The model under review builds one solid part; all positions refer to its coordinate system, in mm. A direction names the side the tool comes from. Round coordinates to 2 decimals unless told otherwise and drop trailing zeros. Write each loop counter-clockwise with the first axis right and the second up, starting at its lowest first coordinate (ties: lowest second). Pieces come first, ordered by that corner, then holes. Notation, with made-up numbers: M 3.5,-28.5 L 42.5,-28.5 A31 ccw 42.5,8.5 Z; hole C 4,32 d7. An arc over 180 degrees is marked long. One line per item, written item: value. Start each with the question number.
1) Wall thickness on probe 1 along Y at (x, z) = (13, 0.8); probe 2 along X at (y, z) = (-21.5, 1.15); probe 3 along Y at (x, z) = (-15, 0.25): over which ranges is each line inside the solid? List them lowest first.
2) For P1, Ø0.6, axis at x = -3.5, z = 1, coming from the -Y side; P2, Ø1, axis at x = -3.5, z = 1, coming from the +Y side, all flat-tipped, find the tip position at first contact; note any pin that passes through.
3) Mouldability with a two-part tool opening along X and no side actions: class faces 1 (the face through (3, -2, 0)), 2 (the face through (-16.55, -6.49, 0.99)), 3 (the face through (22.039, -6.507, 0.986)), 4 (the face through (-4.946, 17.079, 1.014)) as +X half, -X half, draft (parallel to the pull), parting line (faces both ways), or undercut.
4) Take a section at A-A, the plane x = -7.5. Write out the cut boundary in (y, z).
5) Take a section at D-D, the plane x = -15. Write out the cut boundary in (y, z).
6) Tool access review of faces 5 (the face through (9, 16.794, 1)), 6 (the face through (-16.246, 4, 1)), 7 (the face through (9, -21.206, 1)): name each direction out of +Z, -Z, +X, -X, +Y, -Y from which nothing blocks a thin tool from reaching the whole face with its end or side.
7) Take a section at C-C, the plane z = 1.05. State how many separate pieces and enclosed holes the cut face has, and give its area (3 significant figures).
8) Take a section at B-B, the plane x = 20.5. Write out the cut boundary in (y, z).
from build123d import *

# Parameters (mm, degrees)
SKETCH_1_R          = 1
EXTRUDE_4_DEPTH     = 2
FILLET_1_R          = 1
EXTRUDE_5_DEPTH     = 2
SKETCH_5_R          = 1
CUT_EXTRUDE_3_DEPTH = 2
SKETCH_6_W          = 8
SKETCH_6_H          = 3
EXTRUDE_6_DEPTH     = 2


with BuildPart() as part:
    # 草圖1 → 填料-伸長4 (new body)
    with BuildSketch(Plane.XY):
        with BuildLine():
            Line((-19.246232324, 5.793640832), (-17.246232324, 5.793640832))
            ThreePointArc((-17.246232324, 5.793640832), (-16.539125543, 5.500747613), (-16.246232324, 4.793640832))
            Line((-16.246232324, 4.793640832), (-16.246232324, 2.793640832))
            ThreePointArc((-16.246232324, 2.793640832), (-16.539125543, 2.086534051), (-17.246232324, 1.793640832))
            Line((-17.246232324, 1.793640832), (-19.246232324, 1.793640832))
            Line((-19.246232324, 1.793640832), (-19.246232324, -6.206359168))
            Line((-19.246232324, -6.206359168), (-17.246232324, -6.206359168))
            ThreePointArc((-17.246232324, -6.206359168), (-16.539125543, -6.499252387), (-16.246232324, -7.206359168))
            Line((-16.246232324, -7.206359168), (-16.246232324, -9.206359168))
            ThreePointArc((-16.246232324, -9.206359168), (-16.539125543, -9.913465949), (-17.246232324, -10.206359168))
            Line((-17.246232324, -10.206359168), (-19.246232324, -10.206359168))
            Line((-19.246232324, -10.206359168), (-19.246232324, -18.206359168))
            Line((-19.246232324, -18.206359168), (24.753767676, -18.206359168))
            Line((24.753767676, -18.206359168), (24.753767676, -10.206359168))
            Line((24.753767676, -10.206359168), (22.753767676, -10.206359168))
            ThreePointArc((22.753767676, -10.206359168), (22.046660894, -9.913465949), (21.753767676, -9.206359168))
            Line((21.753767676, -9.206359168), (21.753767676, -7.206359168))
            ThreePointArc((21.753767676, -7.206359168), (22.046660894, -6.499252387), (22.753767676, -6.206359168))
            Line((22.753767676, -6.206359168), (24.753767676, -6.206359168))
            Line((24.753767676, -6.206359168), (24.753767676, 1.793640832))
            Line((24.753767676, 1.793640832), (22.753767676, 1.793640832))
            ThreePointArc((22.753767676, 1.793640832), (22.046660894, 2.086534051), (21.753767676, 2.793640832))
            Line((21.753767676, 2.793640832), (21.753767676, 4.793640832))
            ThreePointArc((21.753767676, 4.793640832), (22.046660894, 5.500747613), (22.753767676, 5.793640832))
            Line((22.753767676, 5.793640832), (24.753767676, 5.793640832))
            Line((24.753767676, 5.793640832), (24.753767676, 13.793640832))
            Line((24.753767676, 13.793640832), (-19.246232324, 13.793640832))
            Line((-19.246232324, 13.793640832), (-19.246232324, 5.793640832))
        make_face()
        with Locations((-15.246232324, 7.793640832)):
            Circle(SKETCH_1_R, mode=Mode.SUBTRACT)
        with Locations((-15.246232324, -0.206359168)):
            Circle(SKETCH_1_R, mode=Mode.SUBTRACT)
        with Locations((20.753767676, -12.206359168)):
            Circle(SKETCH_1_R, mode=Mode.SUBTRACT)
        with Locations((20.753767676, 7.793640832)):
            Circle(SKETCH_1_R, mode=Mode.SUBTRACT)
        with Locations((-15.246232324, -4.206359168)):
            Circle(SKETCH_1_R, mode=Mode.SUBTRACT)
        with Locations((-15.246232324, -12.206359168)):
            Circle(SKETCH_1_R, mode=Mode.SUBTRACT)
        with Locations((20.753767676, -0.206359168)):
            Circle(SKETCH_1_R, mode=Mode.SUBTRACT)
        with Locations((20.753767676, -4.206359168)):
            Circle(SKETCH_1_R, mode=Mode.SUBTRACT)
    extrude(amount=EXTRUDE_4_DEPTH)

    # 圓角1
    fillet_1_edges = [part.edges().sort_by_distance(p)[0] for p in [
        (-19.246232324, 13.793640832, 1),
        (24.753767676, 13.793640832, 1),
        (24.753767676, -18.206359168, 1),
        (-19.246232324, -18.206359168, 1),
    ]]
    fillet(fillet_1_edges, radius=FILLET_1_R)

    # 草圖4 → 填料-伸長5 (add)
    with BuildSketch(Plane.XY.offset(2)):
        with BuildLine():
            Line((-19.246232324, -21.206359168), (-19.246232324, -17.206359168))
            Line((-19.246232324, -17.206359168), (24.753767676, -17.206359168))
            Line((24.753767676, -17.206359168), (24.753767676, -21.206359168))
            ThreePointArc((24.753767676, -21.206359168), (24.460874457, -21.913465949), (23.753767676, -22.206359168))
            Line((23.753767676, -22.206359168), (-18.246232324, -22.206359168))
            ThreePointArc((-18.246232324, -22.206359168), (-18.953339106, -21.913465949), (-19.246232324, -21.206359168))
        make_face()
        with BuildLine():
            Line((-19.246232324, 12.793640832), (24.753767676, 12.793640832))
            Line((24.753767676, 12.793640832), (24.753767676, 16.793640832))
            ThreePointArc((24.753767676, 16.793640832), (24.460874457, 17.500747613), (23.753767676, 17.793640832))
            Line((23.753767676, 17.793640832), (-18.246232324, 17.793640832))
            ThreePointArc((-18.246232324, 17.793640832), (-18.953339106, 17.500747613), (-19.246232324, 16.793640832))
            Line((-19.246232324, 16.793640832), (-19.246232324, 12.793640832))
        make_face()
    extrude(amount=-EXTRUDE_5_DEPTH)

    # 草圖5 → 除料-伸長3 (cut)
    with BuildSketch(Plane.XY.offset(2)):
        with Locations(Location((12.753767676, 15.793640832, 0), (0, 0, 180))):
            Circle(SKETCH_5_R)
        with Locations(Location((0.753767676, 15.793640832, 0), (0, 0, 180))):
            Circle(SKETCH_5_R)
        with Locations(Location((0.753767676, -20.206359168, 0), (0, 0, 180))):
            Circle(SKETCH_5_R)
        with Locations(Location((-7.246232324, -20.206359168, 0), (0, 0, 180))):
            Circle(SKETCH_5_R)
        with Locations(Location((4.753767676, -20.206359168, 0), (0, 0, 180))):
            Circle(SKETCH_5_R)
        with Locations(Location((12.753767676, -20.206359168, 0), (0, 0, 180))):
            Circle(SKETCH_5_R)
        with Locations(Location((-7.246232324, 15.793640832, 0), (0, 0, 180))):
            Circle(SKETCH_5_R)
        with Locations(Location((4.753767676, 15.793640832, 0), (0, 0, 180))):
            Circle(SKETCH_5_R)
        with BuildLine():
            Line((-5.246232324, 19.793640832), (-1.246232324, 19.793640832))
            Line((-1.246232324, 19.793640832), (-1.246232324, 17.793640832))
            ThreePointArc((-1.246232324, 17.793640832), (-1.539125543, 17.086534051), (-2.246232324, 16.793640832))
            Line((-2.246232324, 16.793640832), (-4.246232324, 16.793640832))
            ThreePointArc((-4.246232324, 16.793640832), (-4.953339106, 17.086534051), (-5.246232324, 17.793640832))
            Line((-5.246232324, 17.793640832), (-5.246232324, 19.793640832))
        make_face()
        with BuildLine():
            Line((9.753767676, 16.793640832), (7.753767676, 16.793640832))
            ThreePointArc((7.753767676, 16.793640832), (7.046660894, 17.086534051), (6.753767676, 17.793640832))
            Line((6.753767676, 17.793640832), (6.753767676, 19.793640832))
            Line((6.753767676, 19.793640832), (10.753767676, 19.793640832))
            Line((10.753767676, 19.793640832), (10.753767676, 17.793640832))
            ThreePointArc((10.753767676, 17.793640832), (10.460874457, 17.086534051), (9.753767676, 16.793640832))
        make_face()
        with BuildLine():
            Line((10.753767676, -24.206359168), (6.753767676, -24.206359168))
            Line((6.753767676, -24.206359168), (6.753767676, -22.206359168))
            ThreePointArc((6.753767676, -22.206359168), (7.046660894, -21.499252387), (7.753767676, -21.206359168))
            Line((7.753767676, -21.206359168), (9.753767676, -21.206359168))
            ThreePointArc((9.753767676, -21.206359168), (10.460874457, -21.499252387), (10.753767676, -22.206359168))
            Line((10.753767676, -22.206359168), (10.753767676, -24.206359168))
        make_face()
        with BuildLine():
            Line((-4.246232324, -21.206359168), (-2.246232324, -21.206359168))
            ThreePointArc((-2.246232324, -21.206359168), (-1.539125543, -21.499252387), (-1.246232324, -22.206359168))
            Line((-1.246232324, -22.206359168), (-1.246232324, -24.206359168))
            Line((-1.246232324, -24.206359168), (-5.246232324, -24.206359168))
            Line((-5.246232324, -24.206359168), (-5.246232324, -22.206359168))
            ThreePointArc((-5.246232324, -22.206359168), (-4.953339106, -21.499252387), (-4.246232324, -21.206359168))
        make_face()
    extrude(amount=-CUT_EXTRUDE_3_DEPTH, mode=Mode.SUBTRACT)

    # 草圖6 → 填料-伸長6 (add)
    with BuildSketch(Plane.XY.offset(2)):
        Polygon((-19.246232324, -23.206359168), (-19.246232324, -21.206359168), (-5.246232324, -21.206359168), (-5.246232324, -24.206359168), (-18.246232324, -24.206359168), (-19.246232324, -24.206359168), align=None)
        Polygon((-19.246232324, 16.793640832), (-5.246232324, 16.793640832), (-5.246232324, 17.793640832), (-5.246232324, 19.793640832), (-18.246232324, 19.793640832), (-19.246232324, 19.793640832), (-19.246232324, 18.793640832), align=None)
        Polygon((24.753767676, 16.793640832), (24.753767676, 18.793640832), (24.753767676, 19.793640832), (23.753767676, 19.793640832), (10.753767676, 19.793640832), (10.753767676, 16.793640832), align=None)
        Polygon((24.753767676, -21.206359168), (24.753767676, -23.206359168), (24.753767676, -24.206359168), (23.753767676, -24.206359168), (10.753767676, -24.206359168), (10.753767676, -21.206359168), align=None)
        Polygon((-1.246232324, 17.793640832), (-1.246232324, 16.793640832), (6.753767676, 16.793640832), (6.753767676, 19.793640832), (-1.246232324, 19.793640832), align=None)
        with Locations((2.753767676, -22.706359168)):
            Rectangle(SKETCH_6_W, SKETCH_6_H)
    extrude(amount=-EXTRUDE_6_DEPTH)


solid = part.part
Checked values:
1. probe 1: y = -24.21 to -21.18, -19.24 to 14.82, 16.76 to 19.79
1. probe 2: x = -19.25 to -4.95, -1.54 to 7.05, 10.46 to 24.75
1. probe 3: y = -24.21 to -13.18, -11.24 to -5.18, -3.24 to -1.18, 0.76 to 6.82, 8.76 to 19.79
2. P1: stops at y = -21.21
2. P2: stops at y = 16.79
3. face 1: draft
3. face 2: -X half
3. face 3: +X half
3. face 4: undercut
4. outline: M -24.21,0 L -21.17,0 L -21.17,2 L -24.21,2 Z; M -19.24,0 L 14.83,0 L 14.83,2 L -19.24,2 Z; M 16.76,0 L 19.79,0 L 19.79,2 L 16.76,2 Z
5. outline: M -24.21,0 L -13.18,0 L -13.18,2 L -24.21,2 Z; M -11.24,0 L -5.18,0 L -5.18,2 L -11.24,2 Z; M -3.24,0 L -1.18,0 L -1.18,2 L -3.24,2 Z; M 0.76,0 L 6.82,0 L 6.82,2 L 0.76,2 Z; M 8.76,0 L 19.79,0 L 19.79,2 L 8.76,2 Z
6. face 5: +Z, -Z, +Y
6. face 6: +Z, -Z, -X
6. face 7: +Z, -Z, -Y
7. separate pieces: 1
7. enclosed holes: 16
7. area: 1,790 mm2
8. outline: M -24.21,0 L -13.17,0 L -13.17,2 L -24.21,2 Z; M -11.24,0 L -5.17,0 L -5.17,2 L -11.24,2 Z; M -3.24,0 L -1.17,0 L -1.17,2 L -3.24,2 Z; M 0.76,0 L 6.83,0 L 6.83,2 L 0.76,2 Z; M 8.76,0 L 19.79,0 L 19.79,2 L 8.76,2 Z
